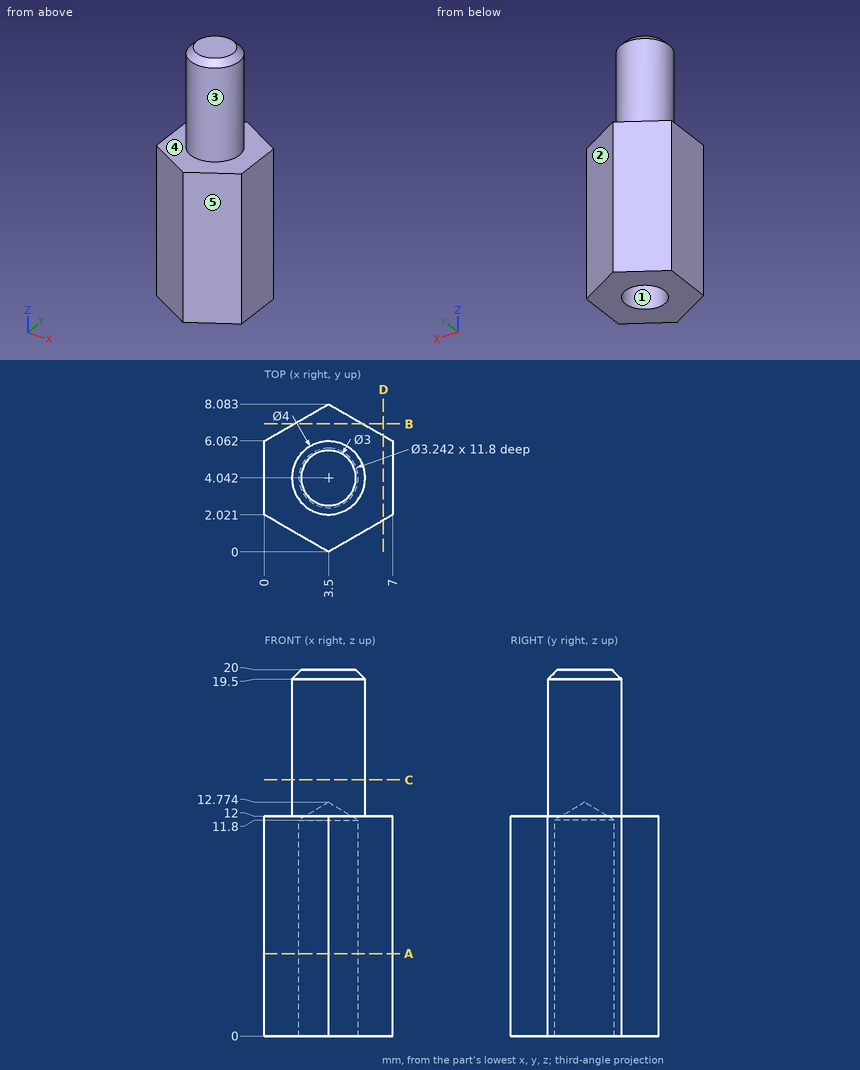
The figure shows three views and two pictorial views of one solid part (mm, origin at its lowest corner). Answer the questions. A direction names the side the tool comes from. Round coordinates to 2 decimals unless told otherwise and drop trailing zeros. Order: outer loops, then holes, each group sorted by start corner. A loop starts at its lowest first (then second) coordinate and runs counter-clockwise, first axis right, second up. Notation, with made-up numbers: M 43,-31 L 88,-31 A25 cw 88,2 Z; hole C -17,-34.75 d7. An arc over 180 degrees is marked long. Answer in a Markdown table with one row per item. Add a question column.
1) The part is cut by section D-D on x = 6.5. Determine the outline of the cut face in (y, z).
2) Consider line 1 along Z through (x, y) = (2, 1.5); line 2 along X through (y, z) = (4, 18.5); line 3 along Y through (x, z) = (2.5, 3.5) (1 decimal). Determine where each line is inside the solid, lowest interval first. Write a range as from..to.
3) Determine the mould class of the marked faces 1, 2 and 3 for opening direction Y: pulls with the +Y half, pulls with the -Y half, needs draft (parallel to the pull), parting line crosses it, or undercut.
4) A flat-ended cylindrical pin translates along its axis: pin 1 Ø1 at (x, z) = (2.5, 4) entering from -Y. Find the tip coordinate at first contact, or state that the pin passes through.
5) Which of the six approach directions +Z, -Z, +X, -X, +Y, -Y give full straight-line access (tool end or side, diameter ignored) to the marked faces 4 and 5?
6) The part is cut by section B-B on y = 7. Determine the outline of the cut face in (x, z) (1 decimal).
7) The part is cut by section C-C on z = 14. Determine the outline of the cut face in (x, y), plus the area to 3 significant figures.
8) The part is cut by section A-A on z = 4.5. Determine the outline of the cut face in (x, y).
Findings below:
| question | item | result |
|---|---|---|
| 1 | outline | M 1.73,0 L 6.35,0 L 6.35,12 L 1.73,12 Z |
| 2 | line 1 | z = 0..12 |
| 2 | line 2 | x = 1.5..5.5 |
| 2 | line 3 | y = 0.6..2.8, 5.3..7.5 |
| 3 | face 1 | undercut |
| 3 | face 2 | pulls with the +Y half |
| 3 | face 3 | parting line crosses it |
| 4 | pin 1 | stops at y = 0.29 |
| 5 | face 4 | +Z |
| 5 | face 5 | +Z, -Z, +X, -Y |
| 6 | outline | M 1.6,0 L 5.4,0 L 5.4,12 L 1.6,12 Z |
| 7 | outline | C 3.5,4.04 d4 |
| 7 | area | 12.6 mm² |
| 8 | outline | M 0,2.02 L 3.5,0 L 7,2.02 L 7,6.06 L 3.5,8.08 L 0,6.06 Z; hole C 3.5,4.04 d3.24 |
